Source: three-view drawing plus pictorial views. Frame: mm from the lowest corner of the part. A direction names the side the tool comes from. Give positions to 0.01 mm unless a question says otherwise; leave off trailing zeros. Write each loop counter-clockwise with the first axis right and the second up, starting at its lowest first coordinate (ties: lowest second). Pieces come first, ordered by that corner, then holes. Notation, with made-up numbers: (-15, -35) -> (-1, -35) arc R12 cw to (-1, -14) -> close; hole circle Ø7 at (-18, -37.5). An arc over 180 degrees is marked (long way). Write item = value, one per line.
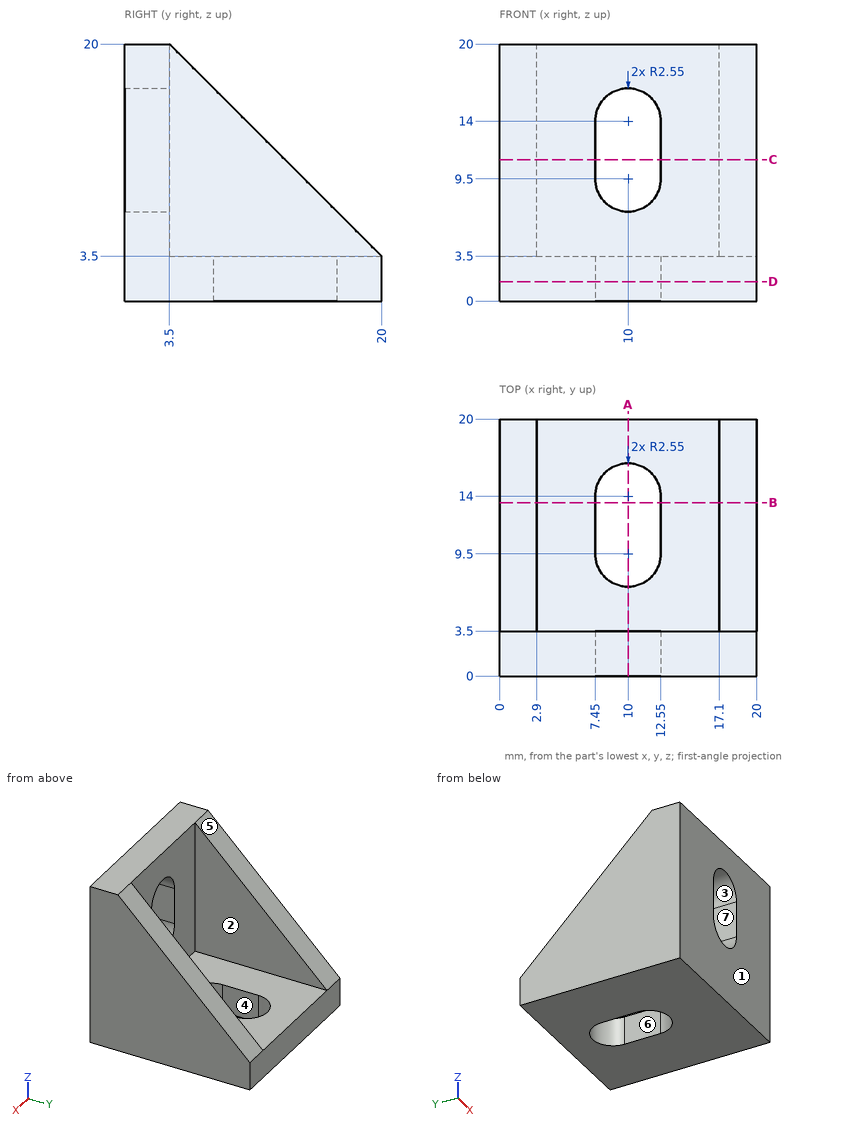
1) Cut plane B-B (y = 13.5). Return the cut outline in (x, z).
Computed:
outline = (0, 0) -> (7.45, 0) -> (7.45, 3.5) -> (2.9, 3.5) -> (2.9, 10) -> (0, 10) -> close; (12.55, 0) -> (20, 0) -> (20, 10) -> (17.1, 10) -> (17.1, 3.5) -> (12.55, 3.5) -> close
2) Contact query for a flat-ended pin moving along its axis: pin 1 (5 mm diameter, centred on x = 14.5, z = 14.5, fed in from +Y). Output: stop coordinate, or through.
Computed:
pin_1 = 3.5
3) Draft query along Y for the marked faces 5, 6 and 7. Return one class per face: pulls with the +Y half, pulls with the -Y half, needs draft (parallel to the pull), parting line crosses it, or undercut.
Computed:
face_5 = pulls with the +Y half
face_6 = undercut
face_7 = needs draft
4) Access query for the marked faces 1, 2, 3 and 4. Directions: +Z, -Z, +X, -X, +Y, -Y. A direction counts if a zero-diameter tool reaches every point of the face in a straight line with its end or side. Return the directions, or none.
Computed:
face_1 = +Z, -Z, +X, -X, -Y
face_2 = +Z, +Y
face_3 = +Y, -Y
face_4 = +Z, -Z
5) Material intervals for L1, parallel to X at y = 8.75, z = 8.5; L2, parallel to X at y = 12, z = 2.75; L3, parallel to Z at x = 4.5, y = 11.75, sorted ascending.
Computed:
L1 = 0 to 2.9, 17.1 to 20
L2 = 0 to 7.45, 12.55 to 20
L3 = 0 to 3.5
6) Cut plane A-A (x = 10). Return the cut outline in (y, z), then the cut area to 4 significant figures.
Computed:
outline = (0, 0) -> (6.95, 0) -> (6.95, 3.5) -> (3.5, 3.5) -> (3.5, 6.95) -> (0, 6.95) -> close; (0, 16.55) -> (3.5, 16.55) -> (3.5, 20) -> (0, 20) -> close; (16.55, 0) -> (20, 0) -> (20, 3.5) -> (16.55, 3.5) -> close
area = 60.55 mm²
7) Cut plane D-D (z = 1.5). Return the cut outline in (x, y), then the cut area to 3 significant figures.
Computed:
outline = (0, 0) -> (20, 0) -> (20, 20) -> (0, 20) -> close; hole (7.45, 9.5) arc R2.55 ccw to (12.55, 9.5) -> (12.55, 14) arc R2.55 ccw to (7.45, 14) -> close
area = 357 mm²
8) Cut plane C-C (z = 11). Return the cut outline in (x, y).
Computed:
outline = (0, 0) -> (7.45, 0) -> (7.45, 3.5) -> (2.9, 3.5) -> (2.9, 12.5) -> (0, 12.5) -> close; (12.55, 0) -> (20, 0) -> (20, 12.5) -> (17.1, 12.5) -> (17.1, 3.5) -> (12.55, 3.5) -> close
